from build123d import *

# Parameters (mm, degrees)
F1_DEPTH = 40
F2_SIZE  = 0.5
F3_SIZE2 = 2.799038
F3_SIZE  = 0.75


with BuildPart() as f1:
    # F0 (on Top) → F1 (new body)
    with BuildSketch(Plane.XY):
        Polygon((-4.5, 4), (-4.5, 0), (4.5, 0), (4.5, 4), (2.75, 4), (2.75, 5), (4.5, 5), (4.5, 6.5), (-4.5, 6.5), (-4.5, 5), (-2.75, 5), (-2.75, 4), align=None)
    extrude(amount=F1_DEPTH)

    # F2
    f2_edges = [f1.edges().sort_by_distance(p)[0] for p in [
        (-4.5, 5, 20),
        (-4.5, 4, 20),
        (4.5, 4, 20),
        (4.5, 5, 20),
        (4.5, 6.5, 20),
        (4.5, 0, 20),
        (-4.5, 6.5, 20),
        (-4.5, 0, 20),
    ]]
    chamfer(f2_edges, length=F2_SIZE)

    # F3
    f3_edges = [f1.edges().sort_by_distance(p)[0] for p in [
        (-2.75, 4.5, 40),
        (2.75, 4.5, 40),
        (-3.375, 4, 40),
        (-3.375, 5, 40),
        (3.375, 5, 40),
        (3.375, 4, 40),
    ]]
    chamfer(f3_edges, length=F3_SIZE, length2=F3_SIZE2)


solid = f1.part
Check sheet for the modelled part. Datum: model origin and axes. Units: mm. A direction names the side the tool comes from. Round coordinates to 2 decimals unless told otherwise and drop trailing zeros. Loops run counter-clockwise (first coordinate to the right, second up) from the corner with the lowest first, then second, coordinate; pieces in that order, holes last. Notation, with made-up numbers: M 84.25,70.25 L 108.25,70.25 A24 ccw 108.25,105.25 Z; hole C -30.75,18 d2. An arc over 180 degrees is marked long. One line per item, written item: value.
(1) Thickness scan on line 1 (Y direction, x = -3, z = 13); line 2 (X direction, y = 4.75, z = 32.5); line 3 (Y direction, x = 4.25, z = 9.5). Record the ranges inside material, lowest first.
Computed values:
line 1: y = 0 to 4, 5 to 6.5
line 2: x = -2.75 to 2.75
line 3: y = 0.25 to 3.75, 5.25 to 6.25
(2) Depth check by flat-ended pin: pin 1 Ø1.1 at (y, z) = (4.5, 16) entering from -X. Enter the tip coordinate at first touch or a pass-through.
Computed values:
pin 1: stops at x = -4.05
(3) Sectioned sample at B-B, the plane z = 16. Record the cut outline in (x, y).
Computed values:
outline: M -4.5,0.5 L -4,0 L 4,0 L 4.5,0.5 L 4.5,3.5 L 4,4 L 2.75,4 L 2.75,5 L 4,5 L 4.5,5.5 L 4.5,6 L 4,6.5 L -4,6.5 L -4.5,6 L -4.5,5.5 L -4,5 L -2.75,5 L -2.75,4 L -4,4 L -4.5,3.5 Z
(4) Sectioned sample at A-A, the plane x = -3.5. Record the cut outline in (y, z), then the cut area to 3 significant figures.
Computed values:
outline: M 0,0 L 4,0 L 4,37.2 L 3.25,40 L 0,40 Z; M 5,0 L 6.5,0 L 6.5,40 L 5.75,40 L 5,37.2 Z
area: 218 mm^2
(5) Sectioned sample at C-C, the plane y = 4.5. Record the cut outline in (x, z).
Computed values:
outline: M -2.75,0 L 2.75,0 L 2.75,37.2 L 2,40 L -2,40 L -2.75,37.2 Z
(6) Access from +Z, -Z, +X, -X, +Y, -Y to the whole of each face (thin tool, end or side, straight path). Record for faces 1 (the face through (-3, 4, 18)), 2 (the face through (-3.268, 5.453, 38.892)), 3 (the face through (3, 5, 18)).
Computed values:
face 1: +Z, -Z, -X
face 2: +Z, -X
face 3: +Z, -Z, +X
(7) Release check for a two-part mould opening along Y. For faces 4 (the face through (4.5, 2, 20)), 5 (the face through (-2.297, 4.518, 38.892)), 6 (the face through (0, 6.5, 20)), 7 (the face through (-3.233, 3.547, 38.892)) record: +Y half, -Y half, draft (parallel to the pull), parting line (faces both ways), or undercut.
Computed values:
face 4: draft
face 5: undercut
face 6: +Y half
face 7: undercut
